The listing builds one solid part. Answer for the finished solid, in the listing's coordinates (mm). A direction names the side the tool comes from. Give positions to 0.01 mm unless a question says otherwise; leave off trailing zeros. Order: outer loops, then holes, each group sorted by start corner. A loop starts at its lowest first (then second) coordinate and runs counter-clockwise, first axis right, second up. Notation, with made-up numbers: (-25, -17) -> (27, -17) arc R28 cw to (27, 7) -> close; hole circle Ø1 at (84, 1.25). An arc over 180 degrees is marked (long way). Answer as a JSON object with one key per item and string values. Group by question number.
```python
from build123d import *

# Parameters (mm, degrees)
SKETCH1_W           = 78.232
SKETCH1_H           = 76.2
BOSS_EXTRUDE1_DEPTH = 35.56
SKETCH2_W           = 75.692
SKETCH2_H           = 73.66
CUT_EXTRUDE1_DEPTH  = 33.02
CUT_EXTRUDE3_DEPTH  = 10.16


with BuildPart() as part:
    # Sketch1 → Boss-Extrude1 (new body)
    with BuildSketch(Plane(origin=(0, 0, 0), x_dir=(1, 0, 0), z_dir=(0, 1, 0))):
        with Locations((39.116, 0)):
            Rectangle(SKETCH1_W, SKETCH1_H)
    extrude(amount=BOSS_EXTRUDE1_DEPTH)

    # Sketch2 → Cut-Extrude1 (cut)
    with BuildSketch(Plane(origin=(0, 35.56, 0), x_dir=(1, 0, 0), z_dir=(0, 1, 0))):
        with Locations((39.116, 0)):
            Rectangle(SKETCH2_W, SKETCH2_H)
    extrude(amount=-CUT_EXTRUDE1_DEPTH, mode=Mode.SUBTRACT)

    # Sketch11 → Cut-Extrude3 (cut)
    with BuildSketch(Plane(origin=(0, 35.56, 0), x_dir=(1, 0, 0), z_dir=(0, 1, 0))):
        Polygon((76.962, -36.83), (76.962, -38.1), (0, -38.1), (0, 38.1), (76.962, 38.1), (76.962, 36.83), (1.27, 36.83), (1.27, -36.83), align=None)
    extrude(amount=-CUT_EXTRUDE3_DEPTH, mode=Mode.SUBTRACT)


solid = part.part
```
(1) A cutting plane is placed at C-C (z = -19). Determine the outline of the cut face in (x, y).
(2) A flat-ended cylindrical pin translates along its axis: pin 1 Ø1.5 at (x, z) = (24, -1.5) entering from +Y. Find the tip coordinate at first contact, or state that the pin passes through.
(3) A cutting plane is placed at A-A (x = 57). Determine the outline of the cut face in (y, z), and give its area (3 significant figures).
(4) Find the intervals of material crossed by line 1 along X through (y, z) = (5.5, -13); line 2 along Z through (x, y) = (54, 14.5); line 3 along Y through (x, z) = (15, 9), in increasing order. Write a range as [from, to].
(5) For a pull along Z with two mould halves and no side action, classify faces 4 (the flat face through (39, 10, -38.1)), 5 (the flat face through (39, 10, 38.1)), 6 (the flat face through (76.962, 19, -1)) as +Z half, -Z half, draft (parallel to the pull), parting line (faces both ways), or undercut.
(6) A cutting plane is placed at D-D (y = 28.5). Determine the outline of the cut face in (x, z).
(7) Which of the six approach directions +Z, -Z, +X, -X, +Y, -Y give full straight-line access (tool end or side, diameter ignored) to faces 1 (the flat face through (39, 14, 36.83)), 2 (the flat face through (39, 25.4, -37)), 3 (the flat face through (78.232, 18, 1))?
(8) A cutting plane is placed at B-B (y = 4). Determine the outline of the cut face in (x, z).
Check sheet entries:
{
 "1": {"outline": "(0, 0) -> (78.23, 0) -> (78.23, 35.56) -> (76.96, 35.56) -> (76.96, 2.54) -> (1.27, 2.54) -> (1.27, 25.4) -> (0, 25.4) -> close"},
 "2": {"pin 1": "stops at y = 2.54"},
 "3": {"outline": "(0, -38.1) -> (25.4, -38.1) -> (25.4, -36.83) -> (2.54, -36.83) -> (2.54, 36.83) -> (25.4, 36.83) -> (25.4, 38.1) -> (0, 38.1) -> close", "area": "252 mm2"},
 "4": {"line 1": "x = [0, 1.27], [76.96, 78.23]", "line 2": "z = [-38.1, -36.83], [36.83, 38.1]", "line 3": "y = [0, 2.54]"},
 "5": {"face 4": "-Z half", "face 5": "+Z half", "face 6": "undercut"},
 "6": {"outline": "(76.96, -38.1) -> (78.23, -38.1) -> (78.23, 38.1) -> (76.96, 38.1) -> close"},
 "7": {"face 1": "+Y", "face 2": "+Z, -Z, -X, +Y", "face 3": "+Z, -Z, +X, +Y, -Y"},
 "8": {"outline": "(0, -38.1) -> (78.23, -38.1) -> (78.23, 38.1) -> (0, 38.1) -> close; hole (1.27, -36.83) -> (76.96, -36.83) -> (76.96, 36.83) -> (1.27, 36.83) -> close"}
}
